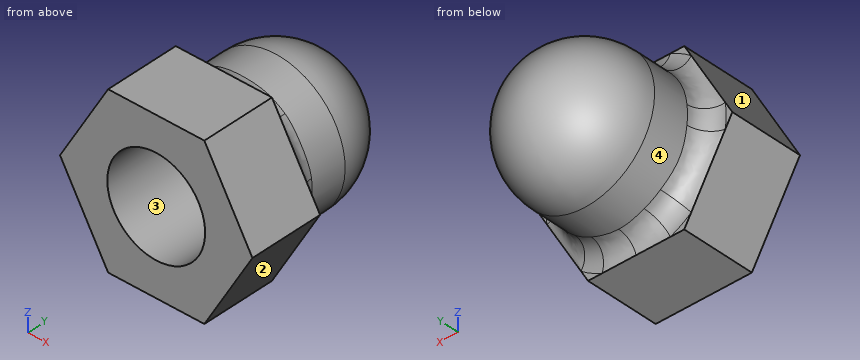
from build123d import *

# Parameters (mm, degrees)
BOSS_EXTRUDE1_DEPTH        = 3.4925
F_12_28_TAPPED_HOLE1_D     = 4.6228
F_12_28_TAPPED_HOLE1_DEPTH = 7.62
F_12_28_TAPPED_HOLE1_TIP   = 0.407562183
FILLET2_R                  = 0.9525


with BuildPart() as part:
    # Sketch1 → Revolve2 (revolve)
    with BuildSketch(Plane.XY, mode=Mode.PRIVATE) as revolve2_sk:
        with BuildLine():
            Line((0, 0), (0, 9.4488))
            ThreePointArc((0, 9.4488), (-2.334866591, 8.481666591), (-3.302, 6.1468))
            Line((-3.302, 6.1468), (-3.302, 0))
            Line((-3.302, 0), (0, 0))
        make_face()
    revolve(revolve2_sk.sketch.rotate(Axis((0, 0, 0), (0, 1, 0)), 270), axis=Axis((0, 0, 0), (0, 1, 0)))

    # Sketch2 → Boss-Extrude1 (add)
    with BuildSketch(Plane.XZ):
        Polygon((4.54605602, 0), (2.27302801, 3.937), (-2.27302801, 3.937), (-4.54605602, 0), (-2.27302801, -3.937), (2.27302801, -3.937), align=None)
    extrude(amount=-BOSS_EXTRUDE1_DEPTH)

    # #12-28 Tapped Hole1
    with Locations(Plane.XZ):
        with Locations((0, 0)):
            Hole(F_12_28_TAPPED_HOLE1_D / 2, depth=F_12_28_TAPPED_HOLE1_DEPTH)
            with Locations((0, 0, -(F_12_28_TAPPED_HOLE1_DEPTH + F_12_28_TAPPED_HOLE1_TIP / 2))):  # 160° drill point
                Cone(0, F_12_28_TAPPED_HOLE1_D / 2, F_12_28_TAPPED_HOLE1_TIP, mode=Mode.SUBTRACT)

    # Fillet2
    fillet2_edges = [part.edges().sort_by_distance(p)[0] for p in [
        (0, 3.4925, 3.302),
    ]]
    fillet(fillet2_edges, radius=FILLET2_R)


solid = part.part
Here's how the part is built. I have some questions about the finished solid (model axes, mm). Face numbers are marked on the shaded views. Coordinates: 2 decimals unless noted, no trailing zeros. Order: outer loops, then holes, each group sorted by start corner. A loop starts at its lowest first (then second) coordinate and runs counter-clockwise, first axis right, second up.
Item 1: I need wall thicknesses on line 1 (Z direction, x = 0, y = 1.5); line 2 (X direction, y = 7.25, z = 0); line 3 (X direction, y = 5.25, z = -1.25). Which ranges of each line are inside material? Lowest first, please.
Result sheet:
line 1: z = -3.94 to -2.31, 2.31 to 3.94
line 2: x = -3.11 to -2.31, 2.31 to 3.11
line 3: x = -3.06 to -1.94, 1.94 to 3.06
Item 2: If we mould it in two halves opening along X, with no side actions, what happens to the marked faces 1, 2, 3 and 4? For each: +X half, -X half, draft (parallel to the pull), parting line (faces both ways), or undercut.
Result sheet:
face 1: -X half
face 2: +X half
face 3: undercut
face 4: parting line
Item 3: If we section it at B-B on y = 7.25: List the corners of the cut face in (x, z) for me, plus the area to 3 significant figures.
Result sheet:
outline: circle Ø6.22 at (0, 0); hole circle Ø4.62 at (0, 0)
area: 13.6 mm2
Item 4: For P1, Ø3, axis at x = -3, z = 0, coming from the +Y side; P2, Ø0.5, axis at x = -2, z = -3.5, coming from the +Y side; P3, Ø2, axis at x = 0.5, y = 7.5, coming from the +Z side, each with a flat end and sliding along its axis, tell me the tip position at first contact or that it passes through.
Result sheet:
P1: stops at y = 9.09
P2: stops at y = 3.62
P3: stops at z = 3.27
Item 5: If we section it at A-A on y = 2: List the corners of the cut face in (x, z) for me, plus the area to 3 significant figures.
Result sheet:
outline: (-4.55, 0) - (-2.27, -3.94) - (2.27, -3.94) - (4.55, 0) - (2.27, 3.94) - (-2.27, 3.94) - close; hole circle Ø4.62 at (0, 0)
area: 36.9 mm2
